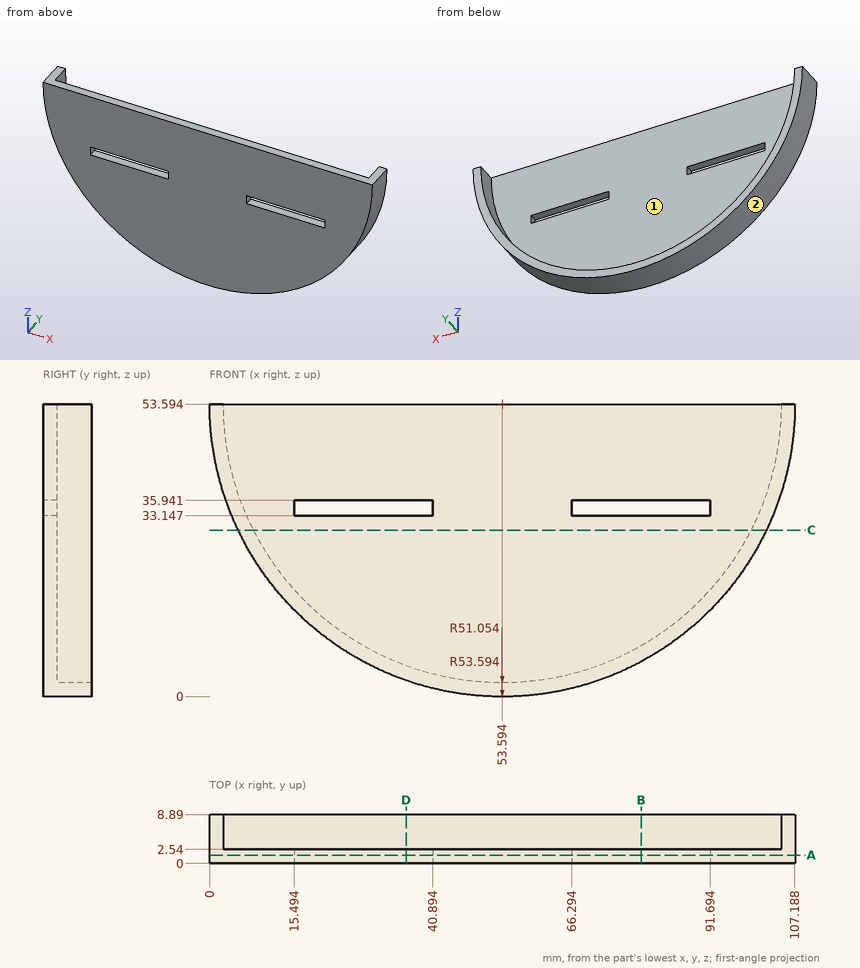
Design review of the part shown in the three views and the two pictorial views. Dimensions are in mm from the part's minimum x, y and z. A direction names the side the tool comes from. Coordinates: 2 decimals unless noted, no trailing zeros. Loops run counter-clockwise (first coordinate to the right, second up) from the corner with the lowest first, then second, coordinate; pieces in that order, holes last. Notation, with made-up numbers: (-13.5, 50) -> (5.5, 50) arc R33 cw to (5.5, 82) -> close; hole circle Ø4 at (40.25, 60). An arc over 180 degrees is marked (long way). Answer as CSV lines item,"result".
Item 1: Take a section at C-C, the plane z = 30.5. State the section outline as (x, y) points, and give its area (3 significant figures).
Results below:
outline,"(5.23, 0) -> (101.96, 0) -> (101.96, 8.89) -> (99.13, 8.89) -> (99.13, 2.54) -> (8.06, 2.54) -> (8.06, 8.89) -> (5.23, 8.89) -> close"
area,"282 mm2"
Item 2: Take a section at A-A, the plane y = 1.5. State the section outline as (x, z) points, and give its area (3 significant figures).
Results below:
outline,"(0, 53.59) arc R53.59 ccw to (107.19, 53.59) -> close; hole (15.49, 33.15) -> (40.89, 33.15) -> (40.89, 35.94) -> (15.49, 35.94) -> close; hole (66.29, 33.15) -> (91.69, 33.15) -> (91.69, 35.94) -> (66.29, 35.94) -> close"
area,"4,370 mm2"
Item 3: Insertion check: pin 1 (1.3 mm diameter, centred on y = 1, z = 34, fed in from +X); pin 2 (3 mm diameter, centred on y = 1, z = 34, fed in from -X); pin 3 (1.3 mm diameter, centred on x = 26.5, y = 1.5, fed in from -Z). Each pin has a flat end and moves straight along its axis. Give the tip position at first contact, or say it passes through.
Results below:
pin 1,"stops at x = 103.73"
pin 2,"stops at x = 3.15"
pin 3,"stops at z = 6.98"
Item 4: For L1, parallel to Y at x = 50, z = 30; L2, parallel to X at y = 4.25, z = 29; L3, parallel to X at y = 8.5, z = 44, list the stretches that pass through material, from the lowest coordinate up.
Results below:
L1,"y = 0 to 2.54"
L2,"x = 5.98 to 8.85, 98.33 to 101.21"
L3,"x = 0.87 to 3.45, 103.74 to 106.32"
Item 5: Machinability: for the marked faces 1 and 2, which of the approach directions +Z, -Z, +X, -X, +Y, -Y give a long, thin tool a straight path to every point of the face, cutting with its end or side? Answer none if there is none.
Results below:
face 1,"+Z, +Y"
face 2,"-Z, +Y, -Y"
Item 6: Take a section at D-D, the plane x = 36. State the section outline as (y, z) points, and give its area (3 significant figures).
Results below:
outline,"(0, 2.97) -> (8.89, 2.97) -> (8.89, 5.67) -> (2.54, 5.67) -> (2.54, 33.15) -> (0, 33.15) -> close; (0, 35.94) -> (2.54, 35.94) -> (2.54, 53.59) -> (0, 53.59) -> close"
area,"139 mm2"
Item 7: Take a section at B-B, the plane x = 79. State the section outline as (y, z) points, and give its area (3 significant figures).
Results below:
outline,"(0, 6.4) -> (8.89, 6.4) -> (8.89, 9.31) -> (2.54, 9.31) -> (2.54, 33.15) -> (0, 33.15) -> close; (0, 35.94) -> (2.54, 35.94) -> (2.54, 53.59) -> (0, 53.59) -> close"
area,"131 mm2"
